For this review, take the finished solid that the model builds, in its own axes (mm). Face numbers are marked on the shaded views. Give positions to 0.01 mm unless a question says otherwise; leave off trailing zeros. Write each loop counter-clockwise with the first axis right and the second up, starting at its lowest first coordinate (ties: lowest second). Pieces come first, ordered by that corner, then holes. Notation, with made-up numbers: M -24.75,-18.75 L -9.75,-18.75 A30 cw -9.75,17.25 Z; hole C 60.25,77 d10. An arc over 180 degrees is marked long. Write item = value, one per line.
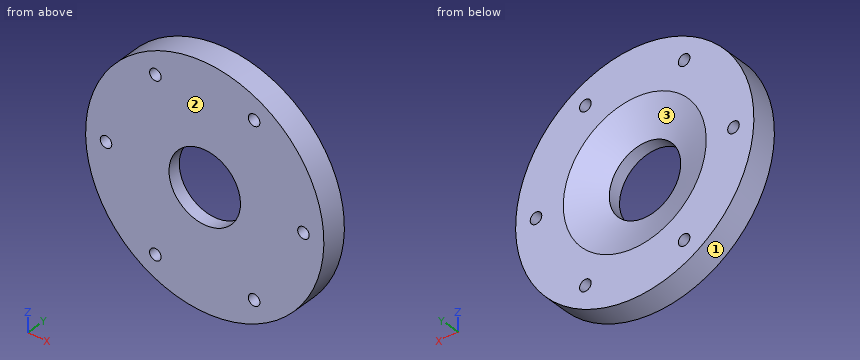
```python
from build123d import *

# Parameters (mm, degrees)
OTW_R_GWINTOWANY_M81_D = 6.8


with BuildPart() as part:
    # Szkic1 → Obrót1 (revolve)
    with BuildSketch(Plane.XY, mode=Mode.PRIVATE) as obr_t1_sk:
        Polygon((-70, 9.103065775), (-70, -5.896934225), (-21, -5.896934225), (-21, 1.603065775), (-42, 9.103065775), align=None)
    revolve(obr_t1_sk.sketch.rotate(Axis((0, 48.980657748, 0), (0, -1, 0)), 270), axis=Axis((0, 48.980657748, 0), (0, -1, 0)))

    # Otwór gwintowany M81 (through all)
    with Locations(Plane(origin=(0, 9.103065775, 0), x_dir=(1, 0, 0), z_dir=(0, 1, 0))):
        with Locations((-58.015165068, 0), (-29.007582534, 50.242606754), (29.007582534, 50.242606754), (58.015165068, 0), (29.007582534, -50.242606754), (-29.007582534, -50.242606754)):
            Hole(OTW_R_GWINTOWANY_M81_D / 2)


solid = part.part
```
1. We need section D-D, the plane x = -48. Write out the cut boundary in (y, z), then the cut area to 3 significant figures.
Responses:
outline = M -5.9,-50.95 L 9.1,-50.95 L 9.1,50.95 L -5.9,50.95 Z
area = 1,530 mm2
2. We need section A-A, the plane x = 0. Write out the cut boundary in (y, z).
Responses:
outline = M -5.9,-70 L 9.1,-70 L 9.1,-42 L 1.6,-21 L -5.9,-21 Z; M -5.9,21 L 1.6,21 L 9.1,42 L 9.1,70 L -5.9,70 Z
3. Insertion check: P1, Ø2, axis at x = 44, y = -2.5, coming from the +Z side; P2, Ø1, axis at x = 14.5, y = 6.5, coming from the +Z side; P3, Ø5, axis at y = -2, z = 40, coming from the -X side; P4, Ø8, axis at x = 29.01, z = 50.24, coming from the -Y side. Each pin has a flat end and moves straight along its axis. Give the tip position at first contact, or say it passes through.
Responses:
P1 = 55.24
P2 = 68.59
P3 = -59.11
P4 = -5.9
4. For line 1 along Z through (x, y) = (31.5, 5); line 2 along Z through (x, y) = (-8, -4); line 3 along Z through (x, y) = (-29, -2.75), list the stretches that pass through material, from the lowest coordinate up. Write a range as from..to.
Responses:
line_1 = -62.51..-52.56, -47.93..47.93, 52.56..62.51
line_2 = -69.54..-19.42, 19.42..69.54
line_3 = -63.71..-53.64, -46.84..46.84, 53.64..63.71
5. The part is to be moulded in two halves that separate along Z. For the marked faces 1, 2 and 3, say which applies: +Z half, -Z half, draft (parallel to the pull), parting line (faces both ways), or undercut.
Responses:
face_1 = parting line
face_2 = draft
face_3 = undercut
6. We need section C-C, the plane y = 0. Write out the cut boundary in (x, z), then the cut area to 3 significant figures.
Responses:
outline = C 0,0 d140; hole C -58.02,0 d6.8; hole C -29.01,-50.24 d6.8; hole C -29.01,50.24 d6.8; hole C 0,0 d42; hole C 29.01,-50.24 d6.8; hole C 29.01,50.24 d6.8; hole C 58.02,0 d6.8
area = 13,800 mm2
7. We need section B-B, the plane z = 0. Write out the cut boundary in (x, y), then the cut area to 3 significant figures.
Responses:
outline = M -70,-5.9 L -61.42,-5.9 L -61.42,9.1 L -70,9.1 Z; M -54.62,-5.9 L -21,-5.9 L -21,1.6 L -42,9.1 L -54.62,9.1 Z; M 21,-5.9 L 54.62,-5.9 L 54.62,9.1 L 42,9.1 L 21,1.6 Z; M 61.42,-5.9 L 70,-5.9 L 70,9.1 L 61.42,9.1 Z
area = 1,110 mm2
